```python
from build123d import *

# Parameters (mm, degrees)
SKETCH_1_R          = 50
EXTRUDE_1_DEPTH     = 5
SKETCH_3_R          = 2.25
CUT_EXTRUDE_1_DEPTH = 3
SKETCH_4_R          = 2.4
CUT_EXTRUDE_2_DEPTH = 3


with BuildPart() as part:
    # Sketch 1 → Extrude 1 (new body)
    with BuildSketch(Plane(origin=(0, 0, 0), x_dir=(1, 0, 0), z_dir=(0, 1, 0))):
        with Locations(Location((0, 0, 0), (0, 0, 270))):
            Circle(SKETCH_1_R)
    extrude(amount=EXTRUDE_1_DEPTH)

    # Sketch 3 → Cut-Extrude 1 (cut)
    with BuildSketch(Plane.XZ):
        with Locations(Location((8, 13.856406461, 0), (0, 0, 270))):
            Circle(SKETCH_3_R)
        with Locations(Location((16, 0, 0), (0, 0, 270))):
            Circle(SKETCH_3_R)
        with Locations(Location((8, -13.856406461, 0), (0, 0, 270))):
            Circle(SKETCH_3_R)
        with Locations(Location((-8, -13.856406461, 0), (0, 0, 270))):
            Circle(SKETCH_3_R)
        with Locations(Location((-16, 0, 0), (0, 0, 270))):
            Circle(SKETCH_3_R)
        with Locations(Location((-8, 13.856406461, 0), (0, 0, 270))):
            Circle(SKETCH_3_R)
    extrude(amount=-CUT_EXTRUDE_1_DEPTH, mode=Mode.SUBTRACT)

    # Sketch 4 → Cut-Extrude 2 (cut)
    with BuildSketch(Plane(origin=(0, 5, 0), x_dir=(1, 0, 0), z_dir=(0, 1, 0))):
        with Locations(Location((0, 40, 0), (0, 0, 270))):
            Circle(SKETCH_4_R)
        with Locations(Location((40, 0, 0), (0, 0, 270))):
            Circle(SKETCH_4_R)
        with Locations(Location((0, -40, 0), (0, 0, 270))):
            Circle(SKETCH_4_R)
        with Locations(Location((-40, 0, 0), (0, 0, 270))):
            Circle(SKETCH_4_R)
    extrude(amount=-CUT_EXTRUDE_2_DEPTH, mode=Mode.SUBTRACT)


solid = part.part
```
Verification items for the finished model (mm, model axes). A direction names the side the tool comes from. Give positions to 0.01 mm unless a question says otherwise; leave off trailing zeros. Loops run counter-clockwise (first coordinate to the right, second up) from the corner with the lowest first, then second, coordinate; pieces in that order, holes last. Notation, with made-up numbers: M 20,9.5 L 38,9.5 A20 ccw 38,23.5 Z; hole C 52,4.25 d4. An arc over 180 degrees is marked long. Return JSON: item names as keys, results as strings.
1) Gauge pin test, flat ends, axial feed: P1, Ø2, axis at x = 35.5, z = -20, coming from the -Y side; P2, Ø4, axis at x = 0, z = -40, coming from the +Y side; P3, Ø1.3, axis at x = 7, z = -14, coming from the -Y side. Record the tip position at first contact, or that the pin passes through.
Findings:
{"P1": "stops at y = 0", "P2": "stops at y = 2", "P3": "stops at y = 3"}
2) Section check C-C, the plane z = 0. Enter the section's corners in (x, y).
Findings:
{"outline": "M -50,0 L -18.25,0 L -18.25,3 L -13.75,3 L -13.75,0 L 13.75,0 L 13.75,3 L 18.25,3 L 18.25,0 L 50,0 L 50,5 L 42.4,5 L 42.4,2 L 37.6,2 L 37.6,5 L -37.6,5 L -37.6,2 L -42.4,2 L -42.4,5 L -50,5 Z"}
3) Tool access check on faces 4 (the flat face through (40, 2, 0)), 5 (the cylindrical face through (-18.196, 1.479, 0.488)). Record the directions out of +Z, -Z, +X, -X, +Y, -Y that give a thin tool (end or side, any length) a straight path to the whole face; none if there is none.
Findings:
{"face 4": "+Y", "face 5": "-Y"}
4) Section check A-A, the plane y = 1.1. Enter the section's corners in (x, z), and give its area (3 significant figures).
Findings:
{"outline": "C 0,0 d100; hole C -16,0 d4.5; hole C -8,-13.86 d4.5; hole C -8,13.86 d4.5; hole C 8,-13.86 d4.5; hole C 8,13.86 d4.5; hole C 16,0 d4.5", "area": "7,760 mm2"}
5) Material ranges on L1, parallel to X at y = 1.6, z = 0; L2, parallel to X at y = 3, z = -38; L3, parallel to Z at x = 36, y = 2.7, recorded low to high. Write a range as [from, to].
Findings:
{"L1": "x = [-50, -18.25], [-13.75, 13.75], [18.25, 50]", "L2": "x = [-32.5, -1.33], [1.33, 32.5]", "L3": "z = [-34.7, 34.7]"}
6) Section check D-D, the plane z = -40. Enter the section's corners in (x, y), and give its area (3 significant figures).
Findings:
{"outline": "M -30,0 L 30,0 L 30,5 L 2.4,5 L 2.4,2 L -2.4,2 L -2.4,5 L -30,5 Z", "area": "286 mm2"}
7) Mould release check, pull along Z, two halves, no side actions. Record for faces 1 (the cylindrical face through (15.02, 2.46, 47.69)), 2 (the cylindrical face through (-42.343, 3.521, -0.52)), 3 (the flat face through (1, 5, -1)): released by +Z, released by -Z, zero draft, split by the parting line, or undercut.
Findings:
{"face 1": "split by the parting line", "face 2": "undercut", "face 3": "zero draft"}
8) Section check B-B, the plane x = -40. Enter the section's corners in (y, z).
Findings:
{"outline": "M 0,-30 L 5,-30 L 5,-2.4 L 2,-2.4 L 2,2.4 L 5,2.4 L 5,30 L 0,30 Z"}
